from build123d import *

# Parameters (mm, degrees)
SKETCH_W     = 149
SKETCH_H     = 149
PAD_DEPTH    = 30
SKETCH001_W  = 143
SKETCH001_H  = 143
POCKET_DEPTH = 27
FILLET_R     = 2
FILLET001_R  = 2


with BuildPart() as part:
    # Sketch → Pad (new body)
    with BuildSketch(Plane.XY):
        Rectangle(SKETCH_W, SKETCH_H)
    extrude(amount=PAD_DEPTH)

    # Sketch001 (on Face6 of Pad) → Pocket (cut)
    with BuildSketch(Plane.XY.offset(30)):
        Rectangle(SKETCH001_W, SKETCH001_H)
    extrude(amount=-POCKET_DEPTH, mode=Mode.SUBTRACT)

    # Fillet
    fillet_edges = [part.edges().sort_by_distance(p)[0] for p in [
        (74.5, -74.5, 15),
        (-74.5, -74.5, 15),
        (74.5, 74.5, 15),
        (-74.5, 74.5, 15),
    ]]
    fillet(fillet_edges, radius=FILLET_R)

    # Fillet001
    fillet001_edges = [part.edges().sort_by_distance(p)[0] for p in [
        (0, 74.5, 0),
        (-74.5, 0, 0),
        (0, -74.5, 0),
        (74.5, 0, 0),
    ]]
    fillet(fillet001_edges, radius=FILLET001_R)


solid = part.part
The listing builds one solid part. Answer for the finished solid, in the listing's coordinates (mm). A direction names the side the tool comes from. Give positions to 0.01 mm unless a question says otherwise; leave off trailing zeros. Write each loop counter-clockwise with the first axis right and the second up, starting at its lowest first coordinate (ties: lowest second). Pieces come first, ordered by that corner, then holes. Notation, with made-up numbers: (-39, 69.5) -> (-25, 69.5) arc R11 cw to (-25, 82.5) -> close; hole circle Ø10 at (35.5, -6.75). An arc over 180 degrees is marked (long way). One line per question, with ' | ' between items. Start each with the question number.
1. Section A-A (y = -11) is taken. Determine the outline of the cut face in (x, z), plus the area to 3 significant figures.
2. Section C-C (z = 26) is taken. Determine the outline of the cut face in (x, y), plus the area to 3 significant figures.
3. For faces 5 (the flat face through (-1, 1, 0)), 6 (the flat face through (-71.5, -1, 17)), determine the directions among +Z, -Z, +X, -X, +Y, -Y from which every point of the face is accessible in a straight line to the end or side of a thin tool.
4. For a pull along Y with two mould halves and no side action, classify faces 1 (the flat face through (-1, -74.5, 16)), 2 (the flat face through (74.5, -1, 16)), 3 (the flat face through (-1, -71.5, 17)), 4 (the flat face through (-1, 1, 3)) as pulls with the +Y half, pulls with the -Y half, needs draft (parallel to the pull), parting line crosses it, or undercut.
5. Find the intervals of material crossed by probe 1 along Y at (x, z) = (-7.5, 14.75); probe 2 along Z at (x, y) = (-56, 36.5), in increasing order.
Response values:
1) outline: (-74.5, 2) arc R2 ccw to (-72.5, 0) -> (72.5, 0) arc R2 ccw to (74.5, 2) -> (74.5, 30) -> (71.5, 30) -> (71.5, 3) -> (-71.5, 3) -> (-71.5, 30) -> (-74.5, 30) -> close | area: 607 mm2
2) outline: (-74.5, -72.5) arc R2 ccw to (-72.5, -74.5) -> (72.5, -74.5) arc R2 ccw to (74.5, -72.5) -> (74.5, 72.5) arc R2 ccw to (72.5, 74.5) -> (-72.5, 74.5) arc R2 ccw to (-74.5, 72.5) -> close; hole (-71.5, -71.5) -> (71.5, -71.5) -> (71.5, 71.5) -> (-71.5, 71.5) -> close | area: 1,750 mm2
3) face 5: -Z, +X, -X, +Y, -Y | face 6: +Z
4) face 1: pulls with the -Y half | face 2: needs draft | face 3: undercut | face 4: undercut
5) probe 1: -74.5 to -71.5, 71.5 to 74.5 | probe 2: 0 to 3
